```python
from build123d import *

# Parameters (mm, degrees)
SKETCH_1_W          = 10
SKETCH_1_H          = 10
EXTRUDE_1_DEPTH     = 190
SKETCH_2_R          = 2.1
CUT_EXTRUDE_1_DEPTH = 200
SKETCH_3_R          = 4
CUT_EXTRUDE_2_DEPTH = 191.131533418


with BuildPart() as part:
    # 草图1 → 凸台-拉伸1 (new body)
    with BuildSketch(Plane(origin=(0, 0, 0), x_dir=(1, 0, 0), z_dir=(0, 1, 0))):
        Rectangle(SKETCH_1_W, SKETCH_1_H)
    extrude(amount=EXTRUDE_1_DEPTH)

    # 草图2 → 切除-拉伸1 (cut)
    with BuildSketch(Plane.XY.offset(5)):
        with Locations((0, 10)):
            Circle(SKETCH_2_R)
        with Locations((0, 30)):
            Circle(SKETCH_2_R)
        with Locations((0, 180)):
            Circle(SKETCH_2_R)
        with Locations((0, 160)):
            Circle(SKETCH_2_R)
    extrude(amount=-CUT_EXTRUDE_1_DEPTH, mode=Mode.SUBTRACT)

    # 草图3 → 切除-拉伸2 (cut, through all)
    with BuildSketch(Plane.XZ):
        with Locations(Location((0, 0, 0), (0, 0, 270))):
            Circle(SKETCH_3_R)
    extrude(amount=-CUT_EXTRUDE_2_DEPTH, mode=Mode.SUBTRACT)


solid = part.part
```
Design review of the part built by this model. Coordinates are the model's own, in mm. Coordinates: 2 decimals unless noted, no trailing zeros. Write each loop counter-clockwise with the first axis right and the second up, starting at its lowest first coordinate (ties: lowest second). Pieces come first, ordered by that corner, then holes.
1) Add section C-C (y = 129.5). Write out the cut boundary in (x, z).
2) Add section B-B (z = 0). Write out the cut boundary in (x, y), plus the area to 3 significant figures.
3) Add section A-A (y = 180). Write out the cut boundary in (x, z), plus the area to 3 significant figures.
4) Add section D-D (x = 0). State how many separate pieces and enclosed holes the cut face has, plus the area to 3 significant figures.
5) To check wall thickness, follow L1, parallel to Y at x = 0, z = 4.2; L2, parallel to X at y = 160, z = 4.6; L3, parallel to Z at x = 0, y = 65. State the ranges of each line that lie inside material, in increasing order.
6) Mouldability with a two-part tool opening along X and no side actions: class faces 1 (the flat face through (0, 94, 5)), 2 (the cylindrical face through (2.003, 30.631, 4.391)), 3 (the flat face through (5, 94, 0)) as +X half, -X half, draft (parallel to the pull), parting line (faces both ways), or undercut.
Check result:
1. outline: (-5, -5) - (5, -5) - (5, 5) - (-5, 5) - close; hole circle Ø8 at (0, 0)
2. outline: (-5, 0) - (-4, 0) - (-4, 190) - (-5, 190) - close; (4, 0) - (5, 0) - (5, 190) - (4, 190) - close
2. area: 380 mm2
3. outline: (-5, -5) - (-2.1, -5) - (-2.1, -3.4) arc R4 cw to (-2.1, 3.4) - (-2.1, 5) - (-5, 5) - close; (2.1, -5) - (5, -5) - (5, 5) - (2.1, 5) - (2.1, 3.4) arc R4 cw to (2.1, -3.4) - close
3. area: 39.7 mm2
4. separate pieces: 10
4. enclosed holes: 0
4. area: 346 mm2
5. L1: y = 0 to 7.9, 12.1 to 27.9, 32.1 to 157.9, 162.1 to 177.9, 182.1 to 190
5. L2: x = -5 to -2.1, 2.1 to 5
5. L3: z = -5 to -4, 4 to 5
6. face 1: draft
6. face 2: undercut
6. face 3: +X half
